from build123d import *

# Parameters (mm, degrees)
SKETCH1_W          = 140.25
SKETCH1_H          = 65
SKETCH1_W_2        = 10.5
SKETCH1_H_2        = 5.1
BASE_FLANGE1_DEPTH = 5


# Sheet-metal steps are written as plain solids
with BuildPart() as part:
    # Sketch1 → Base-Flange1 (new body)
    with BuildSketch(Plane(origin=(0, 0, 0), x_dir=(1, 0, 0), z_dir=(0, 1, 0))):
        Rectangle(SKETCH1_W, SKETCH1_H)
        with Locations((-14.875, 10.025)):
            Rectangle(SKETCH1_W_2, SKETCH1_H_2, mode=Mode.SUBTRACT)
        with Locations((43.625, 10.025)):
            Rectangle(SKETCH1_W_2, SKETCH1_H_2, mode=Mode.SUBTRACT)
        with Locations((15.125, -10.025)):
            Rectangle(SKETCH1_W_2, SKETCH1_H_2, mode=Mode.SUBTRACT)
        with Locations((48.625, -10.025)):
            Rectangle(SKETCH1_W_2, SKETCH1_H_2, mode=Mode.SUBTRACT)
    extrude(amount=-BASE_FLANGE1_DEPTH)


solid = part.part
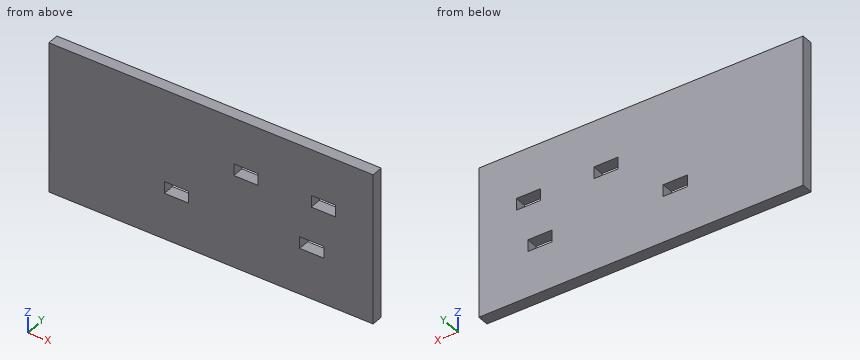
Input: part model. Units: mm. Frame: model coordinates. Coordinates: 2 decimals unless noted, no trailing zeros. Order: outer loops, then holes, each group sorted by start corner. A loop starts at its lowest first (then second) coordinate and runs counter-clockwise, first axis right, second up. Notation, with made-up numbers: M 88.25,50 L 130.25,50 A23 ccw 130.25,86 Z; hole C 83.25,4.5 d10. An arc over 180 degrees is marked long. Answer in a Markdown table with one row per item.
(1) Section query A-A, the plane y = -2.95. Output: boundary loops of the cut face in (x, z) (3 decimals), plus the area to 3 significant figures.
Numbers:
| item | result |
|---|---|
| outline | M -70.125,-32.5 L 70.125,-32.5 L 70.125,32.5 L -70.125,32.5 Z; hole M -20.125,-12.575 L -9.625,-12.575 L -9.625,-7.475 L -20.125,-7.475 Z; hole M 9.875,7.475 L 20.375,7.475 L 20.375,12.575 L 9.875,12.575 Z; hole M 38.375,-12.575 L 48.875,-12.575 L 48.875,-7.475 L 38.375,-7.475 Z; hole M 43.375,7.475 L 53.875,7.475 L 53.875,12.575 L 43.375,12.575 Z |
| area | 8,900 mm^2 |
(2) Material intervals for line 1 (Z direction, x = 48, y = -1.9) (3 decimals); line 2 (Z direction, x = 52.5, y = -2.7) (3 decimals); line 3 (Z direction, x = -19, y = -2) (3 decimals), sorted ascending. Write a range as [from, to].
Numbers:
| item | result |
|---|---|
| line 1 | z = [-32.5, -12.575], [-7.475, 7.475], [12.575, 32.5] |
| line 2 | z = [-32.5, 7.475], [12.575, 32.5] |
| line 3 | z = [-32.5, -12.575], [-7.475, 32.5] |
(3) Section query B-B, the plane z = -9.5. Output: boundary loops of the cut face in (x, y) (3 decimals), plus the area to 3 significant figures.
Numbers:
| item | result |
|---|---|
| outline | M -70.125,-5 L -20.125,-5 L -20.125,0 L -70.125,0 Z; M -9.625,-5 L 38.375,-5 L 38.375,0 L -9.625,0 Z; M 48.875,-5 L 70.125,-5 L 70.125,0 L 48.875,0 Z |
| area | 596 mm^2 |
